Part model, mm, in its own coordinate system. A direction names the side the tool comes from. Coordinates: 2 decimals unless noted, no trailing zeros. Order: outer loops, then holes, each group sorted by start corner. A loop starts at its lowest first (then second) coordinate and runs counter-clockwise, first axis right, second up. Notation, with made-up numbers: M 63,41.5 L 93,41.5 A23 ccw 93,60.5 Z; hole C 76,-26.75 d7. An arc over 180 degrees is marked long. Answer in a Markdown table with one row per item. Add a question column.
from build123d import *

# Parameters (mm, degrees)
EXTRUDE_1_DEPTH          = 14
SKETCH_4_R               = 15.5
EXTRUDE_2_DEPTH          = 5
CUT_EXTRUDE_1_DEPTH      = 182.405486002
CUT_EXTRUDE_1_DEPTH_BACK = 182.405486002
SKETCH_5_R               = 6


with BuildPart() as part:
    # 草图1 → 凸台-拉伸1 (new body)
    with BuildSketch(Plane(origin=(0, 0, 0), x_dir=(0, 0, -1), z_dir=(1, 0, 0))):
        with BuildLine():
            Line((177.445626465, -20), (28.722813233, -20))
            ThreePointArc((28.722813233, -20), (-35, 0), (28.722813233, 20))
            Line((28.722813233, 20), (177.445626465, 20))
            Line((177.445626465, 20), (177.445626465, -20))
        make_face()
    extrude(amount=EXTRUDE_1_DEPTH)

    # 草图4 → 凸台-拉伸2 (add)
    with BuildSketch(Plane(origin=(14, 0, 0), x_dir=(0, 0, -1), z_dir=(1, 0, 0))):
        Circle(SKETCH_4_R)
    extrude(amount=EXTRUDE_2_DEPTH)

    # 草图5 → 切除-拉伸1 (cut, two sides: drawn at the far end of the back side and taken through both)
    with BuildSketch(Plane(origin=(14, 0, 0), x_dir=(0, 0, -1), z_dir=(1, 0, 0)).offset(-CUT_EXTRUDE_1_DEPTH_BACK)):
        with Locations((169.945626465, 12.5)):
            Circle(SKETCH_5_R)
        with Locations((144.945626465, 12.5)):
            Circle(SKETCH_5_R)
        with Locations((144.945626465, -12.5)):
            Circle(SKETCH_5_R)
        with Locations((169.945626465, -12.5)):
            Circle(SKETCH_5_R)
    extrude(amount=CUT_EXTRUDE_1_DEPTH + CUT_EXTRUDE_1_DEPTH_BACK, mode=Mode.SUBTRACT)


solid = part.part
(1) Slice it at A-A (x = 8.5). List the corners of the cut face in (y, z), and give its area (3 significant figures).
(2) Pull direction Z, two halves, no side cores. Call faces 3 (the flat face through (7, 20, -102)), 4 (the flat face through (7, 0, -177.446)), 5 (the cylindrical face through (6.9, -12.24, -163.95)), 6 (the cylindrical face through (16.465, 15.368, 2.018)): pulls with the +Z half, pulls with the -Z half, needs draft (parallel to the pull), parting line crosses it, or undercut.
(3) Slice it at C-C (z = -141). List the corners of the cut face in (x, y).
(4) Wall check: line 1 (Z direction, x = 8, y = -12.5); line 2 (Y direction, x = 12.5, z = -146); line 3 (Z direction, x = 9.5, y = -10). Give the ranges that are in metal, low to high.
(5) Slice it at D-D (y = -12.5). List the corners of the cut face in (x, z), and give its area (3 significant figures).
(6) 3-axis set-ups, long thin cutter, end or side, ignore diameter. For faces 1 (the cylindrical face through (6.902, 8.849, -140.184)), 2 (the flat face through (7, -20, -104)): which of +Z, -Z, +X, -X, +Y, -Y reach the whole face in a straight line?
(7) Slice it at B-B (y = 0). List the corners of the cut face in (x, z).
(8) Drop flat-ended pins along their axis: P1, Ø5, axis at x = 2, z = -131.5, coming from the +Y side; P2, Ø6, axis at x = 15.5, y = -22, coming from the +Z side; P3, Ø5, axis at x = 6, z = -45.5, coming from the -Y side. Give the stop position or say it passes through.
Computed:
| question | item | result |
|---|---|---|
| 1 | outline | M -20,-177.45 L 20,-177.45 L 20,-28.72 A35 ccw long -20,-28.72 Z; hole C -12.5,-169.95 d12; hole C -12.5,-144.95 d12; hole C 12.5,-169.95 d12; hole C 12.5,-144.95 d12 |
| 1 | area | 9,170 mm^2 |
| 2 | face 3 | needs draft |
| 2 | face 4 | pulls with the -Z half |
| 2 | face 5 | undercut |
| 2 | face 6 | parting line crosses it |
| 3 | outline | M 0,-20 L 14,-20 L 14,-17.02 L 0,-17.02 Z; M 0,-7.98 L 14,-7.98 L 14,7.98 L 0,7.98 Z; M 0,17.02 L 14,17.02 L 14,20 L 0,20 Z |
| 4 | line 1 | z = -177.45 to -175.95, -163.95 to -150.95, -138.95 to 32.69 |
| 4 | line 2 | y = -20 to -18.41, -6.59 to 6.59, 18.41 to 20 |
| 4 | line 3 | z = -177.45 to -175.4, -164.49 to -150.4, -139.49 to 33.54 |
| 5 | outline | M 0,-177.45 L 14,-177.45 L 14,-175.95 L 0,-175.95 Z; M 0,-163.95 L 14,-163.95 L 14,-150.95 L 0,-150.95 Z; M 0,-138.95 L 14,-138.95 L 14,-9.17 L 19,-9.17 L 19,9.17 L 14,9.17 L 14,32.69 L 0,32.69 Z |
| 5 | area | 2,700 mm^2 |
| 6 | face 1 | +X, -X |
| 6 | face 2 | -Z, +X, -X, -Y |
| 7 | outline | M 0,-177.45 L 14,-177.45 L 14,-15.5 L 19,-15.5 L 19,15.5 L 14,15.5 L 14,35 L 0,35 Z |
| 8 | P1 | stops at y = 20 |
| 8 | P2 | stops at z = 29.13 |
| 8 | P3 | stops at y = -20 |
